Source: three-view drawing plus pictorial views. Frame: mm from the lowest corner of the part. Round coordinates to 2 decimals unless told otherwise and drop trailing zeros. Write each loop counter-clockwise with the first axis right and the second up, starting at its lowest first coordinate (ties: lowest second). Pieces come first, ordered by that corner, then holes.
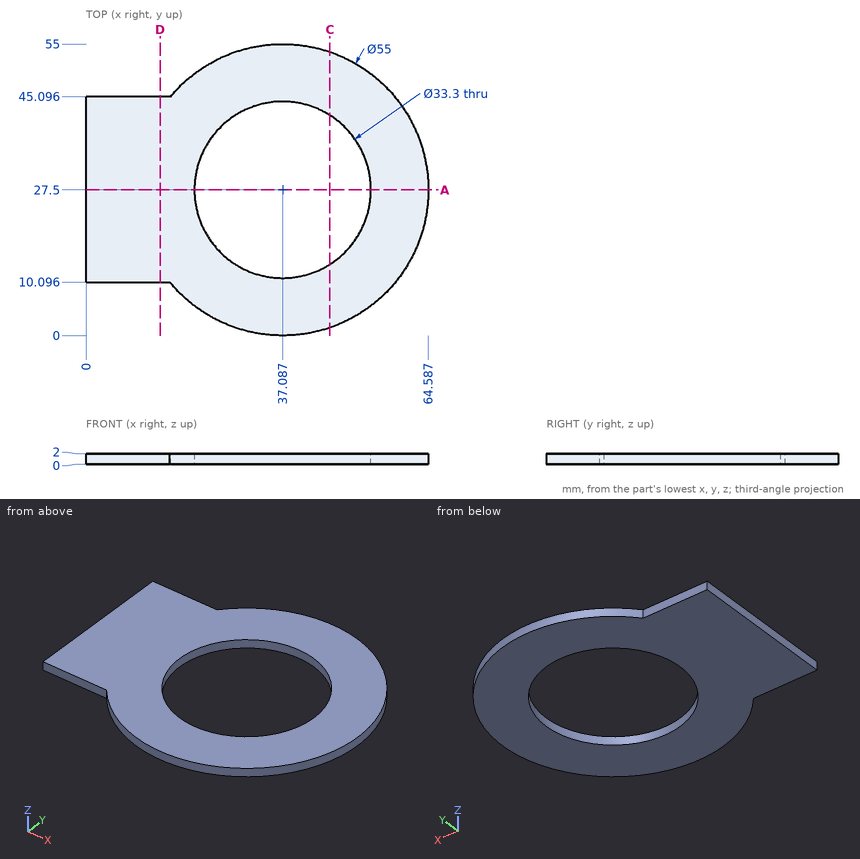
1) Line query: probe 1 along Y at (x, z) = (22, 0.55) (1 decimal); probe 2 along Y at (x, z) = (39.5, 0.95) (1 decimal); probe 3 along X at (y, z) = (39.5, 0.7) (1 decimal). Output: solid intervals per line, ascending.
2) Section D-D on x = 14. Output: boundary loops of the cut face in (y, z) (1 decimal).
3) Section A-A on y = 27.5. Output: boundary loops of the cut face in (x, z).
4) Section C-C on x = 46. Output: boundary loops of the cut face in (y, z) (1 decimal).
5) First-contact query: P1, Ø0.6, axis at x = 10, z = 0.5, coming from the -Y side. Flat tip, straight axial feed; report the tip coordinate or a pass-through.
Filled in:
1. probe 1: y = 4.5 to 20.5, 34.5 to 50.5
1. probe 2: y = 0.1 to 11, 44 to 54.9
1. probe 3: x = 0 to 25.5, 48.6 to 61.8
2. outline: (10.1, 0) - (45.1, 0) - (45.1, 2) - (10.1, 2) - close
3. outline: (0, 0) - (20.44, 0) - (20.44, 2) - (0, 2) - close; (53.74, 0) - (64.59, 0) - (64.59, 2) - (53.74, 2) - close
4. outline: (1.5, 0) - (13.4, 0) - (13.4, 2) - (1.5, 2) - close; (41.6, 0) - (53.5, 0) - (53.5, 2) - (41.6, 2) - close
5. P1: stops at y = 10.1
